Input: part model. Units: mm. Frame: model coordinates. A direction names the side the tool comes from. Give positions to 0.01 mm unless a question says otherwise; leave off trailing zeros. Loops run counter-clockwise (first coordinate to the right, second up) from the corner with the lowest first, then second, coordinate; pieces in that order, holes last. Notation, with made-up numbers: M 4,-24 L 42,-24 A34 ccw 42,11 Z; hole C -2,2 d9. An arc over 180 degrees is marked long. Answer as a JSON object with one key per item and string values. Group by question number.
```python
from build123d import *

# Parameters (mm, degrees)
SKETCH1_W           = 26.289
SKETCH1_H           = 14.224
BOSS_EXTRUDE2_DEPTH = 5.08
BOSS_EXTRUDE3_DEPTH = 5.08
CUT_EXTRUDE1_DEPTH  = 3.4925
CUT_EXTRUDE2_REACH  = 12.16
SKETCH4_R           = 0.3175


with BuildPart() as part:
    # Sketch1 → Boss-Extrude2 (new body)
    with BuildSketch(Plane(origin=(0, 26.595650985, 0), x_dir=(1, 0, 0), z_dir=(0, 1, 0))):
        with Locations((1.874973489, -26.877146351)):
            Rectangle(SKETCH1_W, SKETCH1_H)
    extrude(amount=BOSS_EXTRUDE2_DEPTH)

    # Sketch2 → Boss-Extrude3 (add)
    with BuildSketch(Plane.XZ.offset(-26.595650985)):
        Polygon((-11.269526511, 30.814146351), (-11.269526511, 33.989146351), (15.019473489, 33.989146351), (15.019473489, 30.814146351), (0.858973489, 30.814146351), (0.858973489, 32.401646351), (-4.221026511, 32.401646351), (-4.221026511, 30.814146351), align=None)
    extrude(amount=BOSS_EXTRUDE3_DEPTH)

    # Sketch3 → Cut-Extrude1 (cut)
    with BuildSketch(Plane.XZ.offset(-26.595650985)):
        Polygon((-4.221026511, 30.814146351), (-4.221026511, 32.401646351), (0.858973489, 32.401646351), (0.858973489, 30.814146351), (3.525973489, 30.814146351), (3.525973489, 21.352646351), (-6.888026511, 21.352646351), (-6.888026511, 30.814146351), align=None)
    extrude(amount=-CUT_EXTRUDE1_DEPTH, mode=Mode.SUBTRACT)

    # Sketch4 → Cut-Extrude2 (cut, up to next)
    with BuildSketch(Plane(origin=(0, 31.675650985, 0), x_dir=(1, 0, 0), z_dir=(0, 1, 0)), mode=Mode.PRIVATE) as cut_extrude2_sk1:
        with Locations((5.494473489, -26.908896351)):
            Circle(SKETCH4_R)
    cut_extrude2_tool1 = extrude(cut_extrude2_sk1.sketch, amount=-CUT_EXTRUDE2_REACH, mode=Mode.PRIVATE) & part.part
    add(cut_extrude2_tool1.solids().sort_by_distance((5.494473, 31.675651, 26.908896))[0], mode=Mode.SUBTRACT)
    # Sketch4 → Cut-Extrude2 (cut, up to next)
    with BuildSketch(Plane(origin=(0, 31.675650985, 0), x_dir=(1, 0, 0), z_dir=(0, 1, 0)), mode=Mode.PRIVATE) as cut_extrude2_sk2:
        with Locations((11.844473489, -26.908896351)):
            Circle(SKETCH4_R)
    cut_extrude2_tool2 = extrude(cut_extrude2_sk2.sketch, amount=-CUT_EXTRUDE2_REACH, mode=Mode.PRIVATE) & part.part
    add(cut_extrude2_tool2.solids().sort_by_distance((11.844473, 31.675651, 26.908896))[0], mode=Mode.SUBTRACT)


solid = part.part
```
1. First-contact query: P1, Ø2, axis at y = 25.5, z = 22, coming from the -X side; P2, Ø2, axis at x = -7, y = 24, coming from the -Z side. Flat tips, straight axial feed; report the tip coordinate or a pass-through.
2. Section C-C (z = 22). Output: boundary loops of the cut face in (x, y).
3. Reachability of faces 5 (the flat face through (15.019, 28, 29)), 6 (the flat face through (5, 26.596, 25)), 7 (the flat face through (-2, 28, 21.353)) from +Z, -Z, +X, -X, +Y, -Y: full face, straight path, thin tool, end or side. Return the list, or none.
4. Mould query, pull axis Z, two halves, no side actions, for faces 1 (the flat face through (2, 21.516, 32)), 2 (the flat face through (2, 27, 33.989)), 3 (the flat face through (-2, 30.088, 27)), 4 (the flat face through (3.526, 28, 26)). Classes: pulls with the +Z half, pulls with the -Z half, needs draft (parallel to the pull), parting line crosses it, or undercut.
5. Section D-D (y = 28.25). Output: boundary loops of the cut face in (x, z) (1 decimal).
6. Section A-A (x = 2.75). Output: boundary loops of the cut face in (y, z), then the cut area to 3 significant figures.
7. Section B-B (x = 5.5). Output: boundary loops of the cut face in (y, z).
8. Material intervals for L1, parallel to X at y = 25.5, z = 31; L2, parallel to Z at x = 2.5, y = 28.5; L3, parallel to Z at x = -1.5, y = 27.75, sorted ascending.
Geometry results:
{
 "1": {"P1": "through", "P2": "z = 30.81"},
 "2": {"outline": "M -11.27,26.6 L -6.89,26.6 L -6.89,30.09 L 3.53,30.09 L 3.53,26.6 L 15.02,26.6 L 15.02,31.68 L -11.27,31.68 Z"},
 "3": {"face 5": "+Z, -Z, +X, +Y, -Y", "face 6": "-Z, +X, -X, -Y", "face 7": "-Y"},
 "4": {"face 1": "needs draft", "face 2": "pulls with the +Z half", "face 3": "undercut", "face 4": "undercut"},
 "5": {"outline": "M -11.3,19.8 L 15,19.8 L 15,34 L -11.3,34 Z; hole M -6.9,21.4 L 3.5,21.4 L 3.5,30.8 L 0.9,30.8 L 0.9,32.4 L -4.2,32.4 L -4.2,30.8 L -6.9,30.8 Z; hole C 5.5,26.9 d0.6; hole C 11.8,26.9 d0.6"},
 "6": {"outline": "M 21.52,30.81 L 30.09,30.81 L 30.09,21.35 L 26.6,21.35 L 26.6,19.77 L 31.68,19.77 L 31.68,33.99 L 21.52,33.99 Z", "area": "55.3 mm2"},
 "7": {"outline": "M 21.52,30.81 L 26.6,30.81 L 26.6,27.23 L 31.68,27.23 L 31.68,33.99 L 21.52,33.99 Z; M 26.6,19.77 L 31.68,19.77 L 31.68,26.59 L 26.6,26.59 Z"},
 "8": {"L1": "-11.27 to -4.22, 0.86 to 15.02", "L2": "19.77 to 21.35, 30.81 to 33.99", "L3": "19.77 to 21.35, 32.4 to 33.99"}
}
